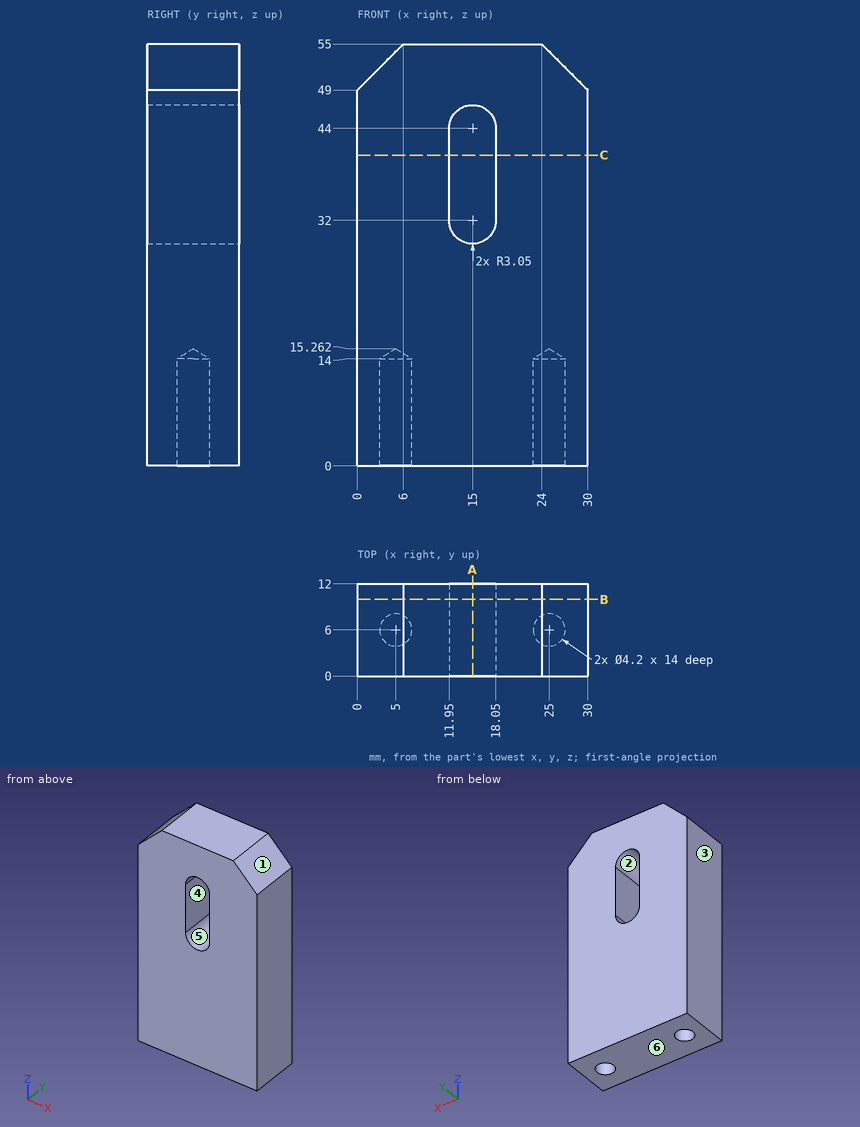
Source: three-view drawing plus pictorial views. Frame: mm from the lowest corner of the part. A direction names the side the tool comes from. Coordinates: 2 decimals unless noted, no trailing zeros. Write each loop counter-clockwise with the first axis right and the second up, starting at its lowest first coordinate (ties: lowest second). Pieces come first, ordered by that corner, then holes. Notation, with made-up numbers: (69.25, 53) - (87.25, 53) arc R25 cw to (87.25, 71) - close; hole circle Ø3 at (69.5, 80.5). An arc over 180 degrees is marked (long way). Answer as a JSON object with one key per item and string values.
Q1. Section query C-C, the plane z = 40.5. Output: boundary loops of the cut face in (x, y), plus the area to 3 significant figures.
Ans:
{"outline": "(0, 0) - (11.95, 0) - (11.95, 12) - (0, 12) - close; (18.05, 0) - (30, 0) - (30, 12) - (18.05, 12) - close", "area": "287 mm2"}
Q2. Section query B-B, the plane y = 10. Output: boundary loops of the cut face in (x, z), plus the area to 3 significant figures.
Ans:
{"outline": "(0, 0) - (30, 0) - (30, 49) - (24, 55) - (6, 55) - (0, 49) - close; hole (11.95, 32) arc R3.05 ccw to (18.05, 32) - (18.05, 44) arc R3.05 ccw to (11.95, 44) - close", "area": "1,510 mm2"}
Q3. Set-up query: the marked faces 1 and 2. Return all of +Z, -Z, +X, -X, +Y, -Y with unobstructed straight access to the full face (end or side cutting, diameter ignored); none if empty.
Ans:
{"face 1": "+Z, +X, +Y, -Y", "face 2": "+Y, -Y"}
Q4. Section query A-A, the plane x = 15. Output: boundary loops of the cut face in (y, z), plus the area to 3 significant figures.
Ans:
{"outline": "(0, 0) - (12, 0) - (12, 28.95) - (0, 28.95) - close; (0, 47.05) - (12, 47.05) - (12, 55) - (0, 55) - close", "area": "443 mm2"}
Q5. Draft query along Z for the marked faces 3, 4, 5 and 6. Return one class per face: released by +Z, released by -Z, zero draft, split by the parting line, or undercut.
Ans:
{"face 3": "zero draft", "face 4": "undercut", "face 5": "undercut", "face 6": "released by -Z"}
Q6. Material intervals for line 1 (Y direction, x = 5, z = 3.5); line 2 (X direction, y = 2.75, z = 36.5); line 3 (Z direction, x = 17, y = 11.25), sorted ascending. Write a range as [from, to].
Ans:
{"line 1": "y = [0, 3.9], [8.1, 12]", "line 2": "x = [0, 11.95], [18.05, 30]", "line 3": "z = [0, 29.7], [46.3, 55]"}
